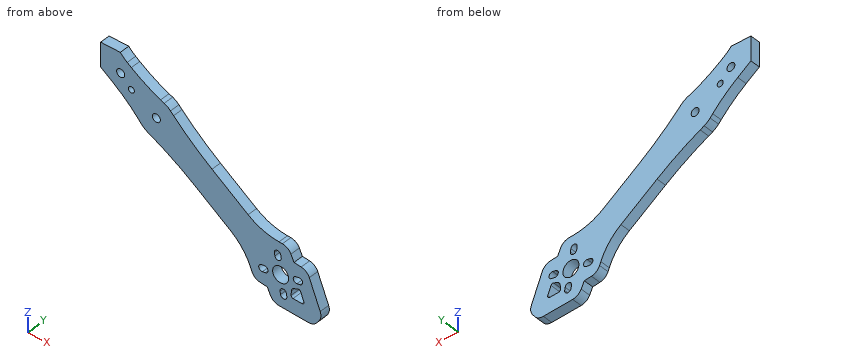
from build123d import *

# Parameters (mm, degrees)
SKETCH2_R           = 2
SKETCH2_R_2         = 1.5
SKETCH2_R_3         = 4
BOSS_EXTRUDE1_DEPTH = 5


with BuildPart() as part:
    # Sketch2 → Boss-Extrude1 (new body)
    with BuildSketch(Plane(origin=(0, 0, 0), x_dir=(1, 0, 0), z_dir=(0, 1, 0))):
        with BuildLine():
            Line((96.674187099, 58.214174471), (100.259554689, 58.62537792))
            ThreePointArc((100.259554689, 58.62537792), (102.726861183, 59.620848143), (104.334258678, 61.740950876))
            Line((104.334258678, 61.740950876), (109.788302134, 75.41951978))
            ThreePointArc((109.788302134, 75.41951978), (110.106786378, 77.879348033), (109.203962948, 80.189563845))
            Line((109.203962948, 80.189563845), (108.148744134, 81.65769437))
            ThreePointArc((108.148744134, 81.65769437), (106.246786582, 83.249782532), (103.813742867, 83.731950064))
            Line((103.813742867, 83.731950064), (89.110198155, 82.922252473))
            ThreePointArc((89.110198155, 82.922252473), (86.58833532, 82.074449344), (84.858361795, 80.053124553))
            Line((84.858361795, 80.053124553), (83.325812901, 76.785825529))
            Line((83.325812901, 76.785825529), (79.745407576, 76.375191199))
            ThreePointArc((79.745407576, 76.375191199), (77.270804519, 75.374131292), (75.6639264, 73.24253003))
            Line((75.6639264, 73.24253003), (75.042843012, 71.6680711))
            ThreePointArc((75.042843012, 71.6680711), (70.946054903, 64.491253119), (64.991367673, 58.761323876))
            Line((64.991367673, 58.761323876), (46.931722679, 45.780954047))
            ThreePointArc((46.931722679, 45.780954047), (36.413241445, 38.843477801), (25.372306119, 32.77184118))
            Line((25.372306119, 32.77184118), (23.401205332, 31.788764494))
            ThreePointArc((23.401205332, 31.788764494), (21.793071121, 30.786042702), (20.402989885, 29.497935256))
            Line((20.402989885, 29.497935256), (19.112268572, 28.051458372))
            ThreePointArc((19.112268572, 28.051458372), (13.16458677, 22.078961314), (6.599736248, 16.792338805))
            Line((6.599736248, 16.792338805), (0, 12.048778377))
            Line((0, 12.048778377), (0, 0))
            Line((0, 0), (9.827416163, 0))
            ThreePointArc((9.827416163, 0), (11.473121255, 1.662110783), (13.293458997, 3.130895317))
            Line((13.293458997, 3.130895317), (15.354276971, 4.612108235))
            ThreePointArc((15.354276971, 4.612108235), (22.457631343, 9.149507995), (30.014371949, 12.883314543))
            Line((30.014371949, 12.883314543), (31.796806607, 13.645668513))
            ThreePointArc((31.796806607, 13.645668513), (33.460801696, 14.552678424), (34.923797775, 15.757331529))
            Line((34.923797775, 15.757331529), (36.483864554, 17.312281519))
            ThreePointArc((36.483864554, 17.312281519), (45.757987001, 25.842092678), (55.686263447, 33.60072351))
            Line((55.686263447, 33.60072351), (73.745908403, 46.581093312))
            ThreePointArc((73.745908403, 46.581093312), (81.074965721, 50.398855458), (89.183263316, 51.994442832))
            Line((89.183263316, 51.994442832), (90.873565855, 52.081292528))
            ThreePointArc((90.873565855, 52.081292528), (93.406161944, 52.924938353), (95.143759302, 54.951397494))
            Line((95.143759302, 54.951397494), (96.674187099, 58.214174471))
        make_face()
        with Locations(Location((10.000016395, 10.000011804, 0), (0, 0, 270))):
            Circle(SKETCH2_R, mode=Mode.SUBTRACT)
        with Locations(Location((27.864354565, 22.840004863, 0), (0, 0, 270))):
            Circle(SKETCH2_R, mode=Mode.SUBTRACT)
        with Locations(Location((15.365, 15.365, 0), (0, 0, 270))):
            Circle(SKETCH2_R_2, mode=Mode.SUBTRACT)
        with Locations(Location((90, 67.5, 0), (0, 0, 270))):
            Circle(SKETCH2_R_3, mode=Mode.SUBTRACT)
        with BuildLine():
            Line((100.618872181, 76.169797692), (96.189048483, 75.92936815))
            ThreePointArc((96.189048483, 75.92936815), (95.498854377, 75.598583427), (95.244713564, 74.876642374))
            Line((95.244713564, 74.876642374), (95.363815249, 72.682238728))
            ThreePointArc((95.363815249, 72.682238728), (95.736845201, 71.623357489), (96.621599456, 70.932278091))
            Line((96.621599456, 70.932278091), (98.663587114, 70.119948739))
            ThreePointArc((98.663587114, 70.119948739), (99.428878121, 70.130724305), (99.962401105, 70.679486242))
            Line((99.962401105, 70.679486242), (101.602243357, 74.8016291))
            ThreePointArc((101.602243357, 74.8016291), (101.485082981, 75.754903393), (100.618872181, 76.169797692))
        make_face(mode=Mode.SUBTRACT)
        with BuildLine():
            Line((99.116926829, 64.38685927), (97.636614954, 64.629092122))
            ThreePointArc((97.636614954, 64.629092122), (96.315997331, 66.466473164), (98.153378372, 67.787090788))
            Line((98.153378372, 67.787090788), (99.633690247, 67.544857936))
            ThreePointArc((99.633690247, 67.544857936), (100.95430787, 65.707476894), (99.116926829, 64.38685927))
        make_face(mode=Mode.SUBTRACT)
        with BuildLine():
            Line((93.11314073, 76.616926829), (92.870907878, 75.136614954))
            ThreePointArc((92.870907878, 75.136614954), (91.033526836, 73.815997331), (89.712909212, 75.653378372))
            Line((89.712909212, 75.653378372), (89.955142064, 77.133690247))
            ThreePointArc((89.955142064, 77.133690247), (91.792523106, 78.45430787), (93.11314073, 76.616926829))
        make_face(mode=Mode.SUBTRACT)
        with BuildLine():
            Line((80.366309753, 67.455142064), (81.846621628, 67.212909212))
            ThreePointArc((81.846621628, 67.212909212), (83.684002669, 68.533526836), (82.363385046, 70.370907878))
            Line((82.363385046, 70.370907878), (80.883073171, 70.61314073))
            ThreePointArc((80.883073171, 70.61314073), (79.04569213, 69.292523106), (80.366309753, 67.455142064))
        make_face(mode=Mode.SUBTRACT)
        with BuildLine():
            Line((90.044857936, 57.866309753), (90.287090788, 59.346621628))
            ThreePointArc((90.287090788, 59.346621628), (88.966473164, 61.184002669), (87.129092122, 59.863385046))
            Line((87.129092122, 59.863385046), (86.88685927, 58.383073171))
            ThreePointArc((86.88685927, 58.383073171), (88.207476894, 56.54569213), (90.044857936, 57.866309753))
        make_face(mode=Mode.SUBTRACT)
    extrude(amount=BOSS_EXTRUDE1_DEPTH)


solid = part.part
Source: CAD feature listing. Evaluate the final solid. Frame: model axes, mm. Give positions to 0.01 mm unless a question says otherwise; leave off trailing zeros. Write each loop counter-clockwise with the first axis right and the second up, starting at its lowest first coordinate (ties: lowest second). Pieces come first, ordered by that corner, then holes. Notation, with made-up numbers: M -15,-32 L 44,-32 A10 cw 44,-26 Z; hole C 70.5,66 d5. An arc over 180 degrees is marked long. Answer as a JSON object with one key per item and string values.
Q1. Contact query for a flat-ended pin moving along its axis: P1, Ø1, axis at y = 3.5, z = -18, coming from the +X side. Output: stop coordinate, or through.
Geometry check:
{"P1": "stops at x = 37.69"}
Q2. Cut plane C-C, the plane y = 2.3. Count the separate pieces of the cut face and the enclosed holes in it, then the cut area to 3 significant figures.
Geometry check:
{"separate pieces": "1", "enclosed holes": "9", "area": "2,180 mm^2"}
Q3. Ray query, line 1 along Z through (x, y) = (91, 2.7); line 2 along Z through (x, y) = (89.5, 1.2); line 3 along X through (y, z) = (1.3, -74). Return the intervals inside material, ascending.
Geometry check:
{"line 1": "z = -83.03 to -78.38, -73.82 to -71.37, -63.63 to -52.09", "line 2": "z = -82.94 to -71.47, -63.53 to -61, -56.9 to -52.01", "line 3": "x = 76.04 to 90.51, 92.08 to 95.29, 101.28 to 109.22"}
Q4. Cut plane A-A, the plane x = 18. Return the cut outline in (y, z).
Geometry check:
{"outline": "M 0,-26.83 L 5,-26.83 L 5,-6.43 L 0,-6.43 Z"}
Q5. Cut plane B-B, the plane z = -43. Return the cut outline in (x, y), then the cut area to 3 significant figures.
Geometry check:
{"outline": "M 42.93,0 L 68.76,0 L 68.76,5 L 42.93,5 Z", "area": "129 mm^2"}
